Read the model definition and answer for the solid it produces. Units are mm, in the model's axes. Face numbers are marked on the shaded views. Coordinates: 2 decimals unless noted, no trailing zeros. Order: outer loops, then holes, each group sorted by start corner. A loop starts at its lowest first (then second) coordinate and runs counter-clockwise, first axis right, second up. Notation, with made-up numbers: (-13.75, 13) -> (36.25, 13) arc R11 cw to (36.25, 23) -> close; hole circle Ø3 at (60, 47). An arc over 180 degrees is marked (long way). Use CSV: the item, a comma, the result in double quotes.
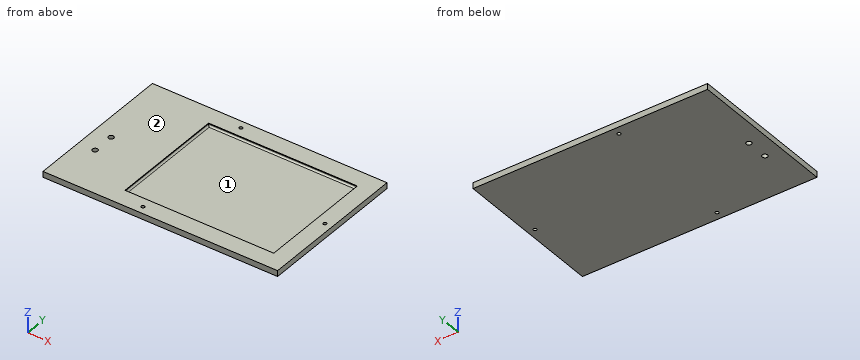
```python
from build123d import *

# Parameters (mm, degrees)
F0_W     = 355.6
F0_H     = 228.6
F1_DEPTH = 8.89
F2_W     = 225.425
F2_H     = 174.625
F3_DEPTH = 3.81
F4_R     = 2.54
F6_D     = 5.1054
F8_D     = 7.9375


with BuildPart() as f1:
    # F0 (on Top) → F1 (new body)
    with BuildSketch(Plane.XY):
        Rectangle(F0_W, F0_H)
    extrude(amount=F1_DEPTH)

    # F2 (on face) → F3 (cut)
    with BuildSketch(Plane.XY.offset(8.89)):
        with Locations((39.6875, 0)):
            Rectangle(F2_W, F2_H)
    extrude(amount=-F3_DEPTH, mode=Mode.SUBTRACT)

    # F4
    f4_edges = [f1.edges().sort_by_distance(p)[0] for p in [
        (39.6875, -87.3125, 5.08),
        (152.4, 0, 5.08),
        (39.6875, 87.3125, 5.08),
        (-73.025, 0, 5.08),
    ]]
    fillet(f4_edges, radius=F4_R)

    # F6 (through all)
    with Locations(Plane.XY.offset(8.89)):
        with Locations((-34.925, -102.39375), (-34.925, 102.39375), (166.6875, 0)):
            Hole(F6_D / 2)

    # F8 (through all)
    with Locations(Plane.XY.offset(8.89)):
        with Locations((-152.4, -7.14375), (-152.4, -40.48125)):
            Hole(F8_D / 2)


solid = f1.part
```
Item 1: This flat-tipped pin is pushed along its axis until it touches: P1, Ø4, axis at x = -35, y = -46.5, coming from the +Z side. Where does it stop, or does it pass through?
Return value:
P1,"stops at z = 5.08"
Item 2: Find section A-A, the plane x = -152.4. Give the number of separate pieces and of enclosed holes in the cut face, then the cut area to 3 significant figures.
Return value:
separate pieces,"3"
enclosed holes,"0"
area,"1,890 mm^2"
Item 3: Find section C-C, the plane x = 76.5. Give the vertices of the cut face in (y, z), then the cut area to 3 significant figures.
Return value:
outline,"(-114.3, 0) -> (114.3, 0) -> (114.3, 8.89) -> (87.31, 8.89) -> (87.31, 7.62) arc R2.54 cw to (84.77, 5.08) -> (-84.77, 5.08) arc R2.54 cw to (-87.31, 7.62) -> (-87.31, 8.89) -> (-114.3, 8.89) -> close"
area,"1,370 mm^2"
Item 4: Straight lines are drawn through the part: line 1 along X through (y, z) = (-78, 7.25); line 2 along Y through (x, z) = (123, 7.5); line 3 along Y through (x, z) = (-153.5, 7.25). For each, find the intervals that lie inside material, in ascending order.
Return value:
line 1,"x = -177.8 to -73, 152.37 to 177.8"
line 2,"y = -114.3 to -87.31, 87.31 to 114.3"
line 3,"y = -114.3 to -44.29, -36.67 to -10.96, -3.33 to 114.3"
Item 5: Find section B-B, the plane y = 74. Give the vertices of the cut face in (x, z) (3 decimals).
Return value:
outline,"(-177.8, 0) -> (177.8, 0) -> (177.8, 8.89) -> (152.4, 8.89) -> (152.4, 7.62) arc R2.54 cw to (149.86, 5.08) -> (-70.485, 5.08) arc R2.54 cw to (-73.025, 7.62) -> (-73.025, 8.89) -> (-177.8, 8.89) -> close"
Item 6: The mould has two halves that part along Y. Classify the marked faces 1 and 2: +Y half, -Y half, draft (parallel to the pull), parting line (faces both ways), or undercut.
Return value:
face 1,"undercut"
face 2,"draft"
